CAD build for the part. Positions are in the model's coordinates, mm. Face numbers are marked on the shaded views. A direction names the side the tool comes from. Give positions to 0.01 mm unless a question says otherwise; leave off trailing zeros. Order: outer loops, then holes, each group sorted by start corner. A loop starts at its lowest first (then second) coordinate and runs counter-clockwise, first axis right, second up. Notation, with made-up numbers: M 71,-28.75 L 109,-28.75 A27 ccw 109,-1.75 Z; hole C 76.5,5.25 d10. An arc over 180 degrees is marked long. Put each result on its own line as item: value. Start each with the question number.
1) Cut at D-D (z = 13.25). Write the cut outline in (x, y).
2) Cut at A-A (y = 0). Write the cut outline in (x, z).
3) Tool access for the marked faces 1 and 2: list every direction of +Z, -Z, +X, -X, +Y, -Y with a clear straight run to the whole face (end or side of a thin tool).
4) Pin check, flat tip, straight feed: pin 1 (3 mm diameter, centred on y = -0.5, z = 4, fed in from +X). Stop position of the tip, or through.
5) Drill centre lines: line 1 (Y direction, x = -0.1, z = 12.5); line 2 (Y direction, x = -1.3, z = 9.25); line 3 (X direction, y = 0.2, z = 6.25). Where is each one in solid material? Low to high. Write a range as [from, to].
6) Cut at C-C (z = 6). Write the cut outline in (x, y).
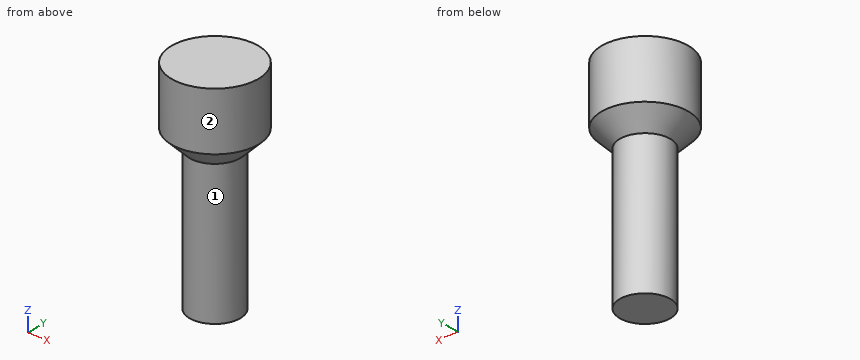
```python
from build123d import *

# Parameters (mm, degrees)
CYLINDER_R        = 1.75
CYLINDER_DEPTH    = 10
CYLINDER001_R     = 3
CYLINDER001_DEPTH = 4


with BuildPart() as screw_cone:
    # Cone → Cone (revolve)
    with BuildSketch(Plane(origin=(0, 0, 9), x_dir=(1, 0, 0), z_dir=(0, -1, 0))):
        Polygon((0, 0), (1, 0), (3, 2), (0, 2), align=None)
    revolve(axis=Axis((0, 0, 9), (0, 0, 1)))


with BuildPart() as screw_cylinder:
    # Cylinder → Cylinder (new body)
    with BuildSketch(Plane.XY):
        Circle(CYLINDER_R)
    extrude(amount=CYLINDER_DEPTH)


with BuildPart() as screw_fusion:
    # Cylinder001 → Cylinder001 (new body)
    with BuildSketch(Plane.XY.offset(11)):
        Circle(CYLINDER001_R)
    extrude(amount=CYLINDER001_DEPTH)

    # Fusion: union screw-cone, screw-cylinder
    add(screw_cone.part)
    add(screw_cylinder.part)


solid = screw_fusion.part
```
Solution:
1. outline: C 0,0 d6
2. outline: M -3,11 L -1.75,9.75 L -1.75,0 L 1.75,0 L 1.75,9.75 L 3,11 L 3,15 L -3,15 Z
3. face 1: -Z
3. face 2: +Z, -Z
4. pin 1: x = 1.75
5. line 1: [-3, 3]
5. line 2: [-1.17, 1.17]
5. line 3: [-1.74, 1.74]
6. outline: C 0,0 d3.5
